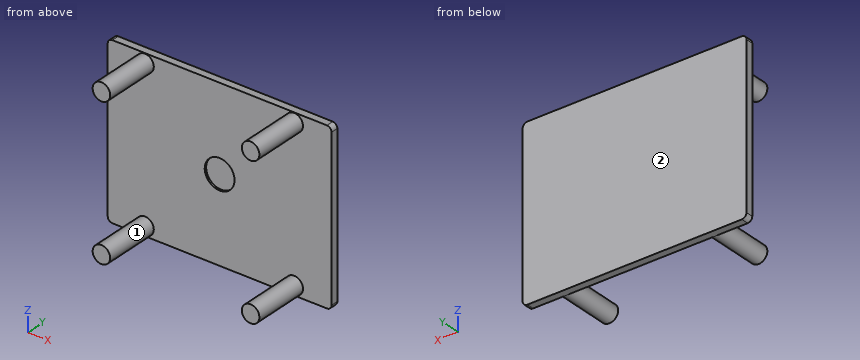
Autodesk Inventor part; units mm, degrees
ref_plane "YZ Plane" through (0, 0, 0) normal (1, 0, 0) x (0, 1, 0)
ref_plane "XZ Plane" through (0, 0, 0) normal (0, 1, 0) x (-1, 0, 0)
ref_plane "XY Plane" through (0, 0, 0) normal (0, 0, 1) x (1, 0, 0)
sketch "Sketch2" plane through (0, 0, 0) normal (0, 1, 0) x (-1, 0, 0)
  line L0 (-60, 60) -> (60, 60)
  line L1 (60, 60) -> (60, -60)
  line L2 (60, -60) -> (-60, -60)
  line L3 (-60, -60) -> (-60, 60)
  line L4 (-60, 60) -> (60, -60) construction
  line L5 (60, 60) -> (-60, -60) construction
  point P0 (0, 0)
  dimension "d4" = 120
  dimension "d5" = 120
extrude "Extrusion2" add sketch "Sketch2" along normal blind 4
sketch "Sketch3" plane through (0, 0, 0) normal (0, -1, 0) x (1, 0, 0)
  line L0 (-40, 40) -> (40, 40) construction
  line L1 (40, 40) -> (40, -40) construction
  line L2 (40, -40) -> (-40, -40) construction
  line L3 (-40, -40) -> (-40, 40) construction
  line L4 (-40, 40) -> (40, -40) construction
  line L5 (40, 40) -> (-40, -40) construction
  circle A0 centre (40, 40) radius 4.7
  circle A1 centre (-40, 40) radius 4.7
  circle A2 centre (-40, -40) radius 4.7
  circle A3 centre (40, -40) radius 4.7
  point P0 (0, 0)
  dimension "d8" = 80
  dimension "d9" = 80
  dimension "d10" = 9.4
  dimension "d13" = 360
extrude "Extrusion3" add sketch "Sketch3" along normal blind 30
sketch "Sketch4" plane through (0, 0, 0) normal (0, -1, 0) x (1, 0, 0)
  point P0 (0, 0)
  point P1 (0, 0)
hole "Hole1" at (0, 0, 0) direction (0, 1, 0) diameter 16 depth 1
sketch "Sketch5" plane through (0, 4, 0) normal (0, 1, 0) x (1, 0, 0)
  line L0 (60, -60) -> (60, 60)
  line L1 (-60, -60) -> (60, -60)
  line L2 (60, -60) -> (60, -45)
  line L3 (60, -45) -> (-60, -45)
  line L4 (-60, -45) -> (-60, -60)
  line L5 (60, 60) -> (-60, 60)
  line L6 (-60, 60) -> (60, 60)
  line L7 (60, 60) -> (60, 45)
  line L8 (60, 45) -> (-60, 45)
  line L9 (-60, 45) -> (-60, 60)
  point P0 (0, 0)
  dimension "d24" = 15
  dimension "d25" = 15
extrude "Extrusion4" cut sketch "Sketch5" against normal up to surface (4 mm away)
fillet "Fillet2" radius 2.5 4 edges at (60, 2, 45) (60, 2, -45) (-60, 2, 45) (-60, 2, -45)
properties part number "sliding_surface_3DPrint"
Geometry: final body of the model. Coordinates: model frame, mm. Face numbers are marked on the shaded views. Round coordinates to 2 decimals unless told otherwise and drop trailing zeros. Loops run counter-clockwise (first coordinate to the right, second up) from the corner with the lowest first, then second, coordinate; pieces in that order, holes last.
Q1. Section B-B on z = 0. Return loops of the section in (x, y), plus the area to 3 significant figures.
Q2. Section D-D on x = 40. Return loops of the section in (y, z), plus the area to 3 significant figures.
Q3. Material intervals for L1, parallel to X at y = 0.5, z = 0; L2, parallel to Z at x = 0, y = 0.4; L3, parallel to Y at x = 29.5, z = 12.5, sorted ascending.
Q4. Pull-direction query (Z, two-part tool) for the marked faces 1 and 2; classes: released by +Z, released by -Z, zero draft, split by the parting line, or undercut.
Q5. Section C-C on x = 0. Return loops of the section in (y, z).
Q6. Pin query (flat end, axial travel): P1, Ø1, axis at x = 0, z = -32, coming from the -Y side; P2, Ø1, axis at x = 42.5, y = -7.5, coming from the +Z side; P3, Ø13, axis at x = 0, z = 0, coming from the -Y side. Return the tip coordinate at first contact, or that it passes through.
Q7. Section A-A on y = -18.5. Return loops of the section in (x, z), plus the area to 3 significant figures.
Evaluation:
1. outline: (-60, 0) - (-8, 0) - (-8, 1) - (8, 1) - (8, 0) - (60, 0) - (60, 4) - (-60, 4) - close
1. area: 464 mm2
2. outline: (-30, -44.7) - (0, -44.7) - (0, -45) - (4, -45) - (4, 45) - (0, 45) - (0, 44.7) - (-30, 44.7) - (-30, 35.3) - (0, 35.3) - (0, -35.3) - (-30, -35.3) - close
2. area: 924 mm2
3. L1: x = -60 to -8, 8 to 60
3. L2: z = -45 to -8, 8 to 45
3. L3: y = 0 to 4
4. face 1: undercut
4. face 2: zero draft
5. outline: (0, -45) - (4, -45) - (4, 45) - (0, 45) - (0, 8) - (1, 8) - (1, -8) - (0, -8) - close
6. P1: stops at y = 0
6. P2: stops at z = 44.25
6. P3: stops at y = 1
7. outline: circle Ø9.4 at (-40, -40); circle Ø9.4 at (-40, 40); circle Ø9.4 at (40, -40); circle Ø9.4 at (40, 40)
7. area: 278 mm2
